Input: part model. Units: mm. Frame: model coordinates. Coordinates: 2 decimals unless noted, no trailing zeros. Order: outer loops, then holes, each group sorted by start corner. A loop starts at its lowest first (then second) coordinate and runs counter-clockwise, first axis right, second up. Notation, with made-up numbers: M 41.25,32.25 L 67.25,32.25 A21 cw 67.25,40.25 Z; hole C 49,13.5 d9. An arc over 180 degrees is marked long. Answer in a Markdown table with one row per item.
from build123d import *

# Parameters (mm, degrees)
SKETCH1_R           = 90
SKETCH1_R_2         = 3
BOSS_EXTRUDE1_DEPTH = 2


with BuildPart() as part:
    # Sketch1 → Boss-Extrude1 (new body)
    with BuildSketch(Plane(origin=(0, 0, 0), x_dir=(1, 0, 0), z_dir=(0, 1, 0))):
        Circle(SKETCH1_R)
        Circle(SKETCH1_R_2, mode=Mode.SUBTRACT)
        with Locations((0, 80)):
            Circle(SKETCH1_R_2, mode=Mode.SUBTRACT)
        with Locations((56.568542495, 56.568542495)):
            Circle(SKETCH1_R_2, mode=Mode.SUBTRACT)
        with Locations((80, 0)):
            Circle(SKETCH1_R_2, mode=Mode.SUBTRACT)
        with Locations((56.568542495, -56.568542495)):
            Circle(SKETCH1_R_2, mode=Mode.SUBTRACT)
        with Locations((0, -80)):
            Circle(SKETCH1_R_2, mode=Mode.SUBTRACT)
        with Locations((-56.568542495, -56.568542495)):
            Circle(SKETCH1_R_2, mode=Mode.SUBTRACT)
        with Locations((-80, 0)):
            Circle(SKETCH1_R_2, mode=Mode.SUBTRACT)
        with Locations((-56.568542495, 56.568542495)):
            Circle(SKETCH1_R_2, mode=Mode.SUBTRACT)
    extrude(amount=BOSS_EXTRUDE1_DEPTH)


solid = part.part
1) Material intervals for probe 1 along Z at (x, y) = (0, 0.8); probe 2 along X at (y, z) = (0.95, 1.5), sorted ascending.
Resolved:
| item | result |
|---|---|
| probe 1 | z = -90 to -83, -77 to -3, 3 to 77, 83 to 90 |
| probe 2 | x = -89.99 to -82.6, -77.4 to -2.6, 2.6 to 77.4, 82.6 to 89.99 |
2) Cut plane A-A, the plane x = 0. Output: boundary loops of the cut face in (y, z).
Resolved:
| item | result |
|---|---|
| outline | M 0,-90 L 2,-90 L 2,-83 L 0,-83 Z; M 0,-77 L 2,-77 L 2,-3 L 0,-3 Z; M 0,3 L 2,3 L 2,77 L 0,77 Z; M 0,83 L 2,83 L 2,90 L 0,90 Z |
3) Cut plane C-C, the plane z = 80. Output: boundary loops of the cut face in (x, y).
Resolved:
| item | result |
|---|---|
| outline | M -41.23,0 L -3,0 L -3,2 L -41.23,2 Z; M 3,0 L 41.23,0 L 41.23,2 L 3,2 Z |
4) Cut plane D-D, the plane y = 1.1. State how many separate pieces and enclosed holes the cut face has, and give its area (3 significant figures).
Resolved:
| item | result |
|---|---|
| separate pieces | 1 |
| enclosed holes | 9 |
| area | 25,200 mm2 |
5) Cut plane B-B, the plane x = -80. Output: boundary loops of the cut face in (y, z).
Resolved:
| item | result |
|---|---|
| outline | M 0,-41.23 L 2,-41.23 L 2,-3 L 0,-3 Z; M 0,3 L 2,3 L 2,41.23 L 0,41.23 Z |
6) Contact query for flat-ended pins moving along their axis: pin 1 (1 mm diameter, centred on y = 1.5, z = 59, fed in from -X); pin 2 (3.5 mm diameter, centred on x = -56.57, z = -56.57, fed in from -Y); pin 3 (1 mm diameter, centred on y = 0.5, z = -13.5, fed in from +X); pin 4 (1 mm diameter, centred on x = 67, y = 1.5, fed in from +Z). Output: stop coordinate, or through.
Resolved:
| item | result |
|---|---|
| pin 1 | stops at x = -68.39 |
| pin 2 | passes through |
| pin 3 | stops at x = 89.06 |
| pin 4 | stops at z = 60.64 |
